Study the drawing (mm; zero at the part's minimum x, y, z) and answer. A direction names the side the tool comes from. Coordinates: 2 decimals unless noted, no trailing zeros. Loops run counter-clockwise (first coordinate to the right, second up) from the corner with the lowest first, then second, coordinate; pieces in that order, holes last. Notation, with made-up numbers: (-29.75, -15.5) -> (-18.75, -15.5) arc R13 cw to (-18.75, -1.5) -> close; hole circle Ø11 at (-38.75, 7). An arc over 180 degrees is marked (long way). Answer as a JSON object with one key per item and string values. Group by question number.
Q1. For the marked faces 1 and 2, determine the directions among +Z, -Z, +X, -X, +Y, -Y from which every point of the face is accessible in a straight line to the end or side of a thin tool.
Q2. A straight line is drawn through the part: line 1 along Y through (x, z) = (6.5, 0.5). Find the intervals that lie inside material, in ascending order. Write a range as [from, to].
Q3. The part is cut by section A-A on y = 5. Write down the section's boundary in (x, z).
Q4. Each of these flat-tipped pins is pushed along its axis until it touches: P1, Ø3, axis at x = 8.5, z = 4, coming from the -Y side; P2, Ø2.5, axis at x = 4.5, y = 4, coming from the -Z side; P3, Ø2.5, axis at x = 3, z = 2.5, coming from the -Y side; P4, Ø5, axis at y = 5, z = 2.5, coming from the -X side. Where does it stop, or does it pass through?
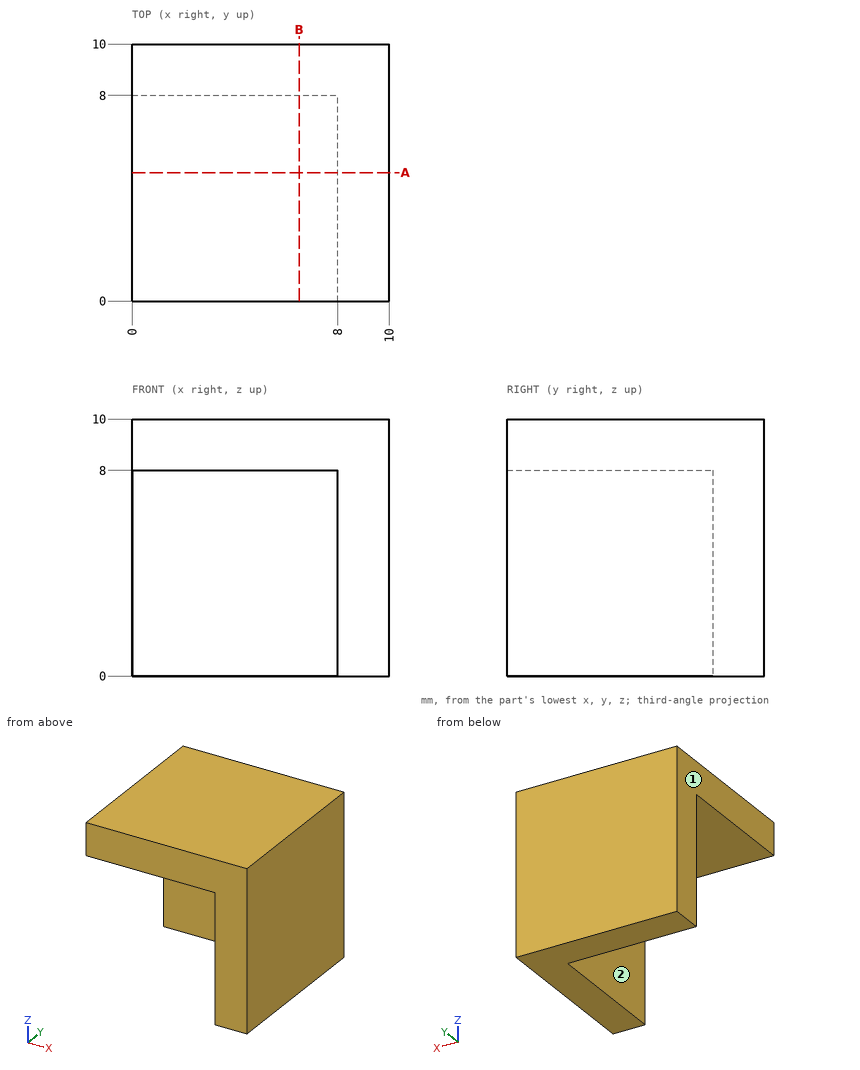
Final values:
{
 "1": {"face 1": "+Z, -Z, -X, +Y, -Y", "face 2": "-Z, -X, -Y"},
 "2": {"line 1": "y = [8, 10]"},
 "3": {"outline": "(0, 8) -> (8, 8) -> (8, 0) -> (10, 0) -> (10, 10) -> (0, 10) -> close"},
 "4": {"P1": "stops at y = 0", "P2": "stops at z = 8", "P3": "stops at y = 8", "P4": "stops at x = 8"}
}
